from build123d import *

# Parameters (mm, degrees)
EXTRUSION1_DEPTH        = 21
ESQUISSE2_R             = 2.5
ENL_V_MAT_EXTRU_1_DEPTH = 22
ESQUISSE3_R             = 2.5
ENL_V_MAT_EXTRU_2_DEPTH = 40.5


with BuildPart() as part:
    # Esquisse1 → Extrusion1 (new body)
    with BuildSketch(Plane.XY):
        Polygon((0, -10.5), (0, 10.5), (9, 10.5), (9, 29), (34, 29), (34, 20), (14, 20), (14, -20), (34, -20), (34, -29), (9, -29), (9, -10.5), align=None)
    extrude(amount=EXTRUSION1_DEPTH)

    # Esquisse2 → Enlèv. mat.-Extru.1 (cut, through all)
    with BuildSketch(Plane.XY.offset(21)):
        with Locations((29, 24.5)):
            Circle(ESQUISSE2_R)
        with Locations((19, 24.5)):
            Circle(ESQUISSE2_R)
        with Locations((19, -24.5)):
            Circle(ESQUISSE2_R)
        with Locations((29, -24.5)):
            Circle(ESQUISSE2_R)
    extrude(amount=-ENL_V_MAT_EXTRU_1_DEPTH, mode=Mode.SUBTRACT)

    # Esquisse3 → Enlèv. mat.-Extru.2 (cut, through all)
    with BuildSketch(Plane(origin=(0, 10.5, 0), x_dir=(1, 0, 0), z_dir=(0, 1, 0))):
        with Locations((4.5, -5.5)):
            Circle(ESQUISSE3_R)
        with Locations((4.5, -15.5)):
            Circle(ESQUISSE3_R)
    extrude(amount=-ENL_V_MAT_EXTRU_2_DEPTH, mode=Mode.SUBTRACT)


solid = part.part
Could you check a few things on this model? Use its own coordinates, in mm. A direction names the side the tool comes from. Coordinates: 2 decimals unless noted, no trailing zeros. Loops run counter-clockwise (first coordinate to the right, second up) from the corner with the lowest first, then second, coordinate; pieces in that order, holes last. Notation, with made-up numbers: (-27, 9.5) -> (-8, 9.5) arc R19 ccw to (-8, 46.5) -> close; hole circle Ø6 at (49.5, -38). An arc over 180 degrees is marked (long way). Answer in a Markdown table with one row per item.
(1) For faces 5 (the face through (5, -10.5, 10)), 6 (the face through (4, 10.5, 10)), 7 (the face through (14, 0, 10)), which set-ups out of +Z, -Z, +X, -X, +Y, -Y let a thin tool reach every point of the face, with its end or its side?
Results found:
| item | result |
|---|---|
| face 5 | +Z, -Z, -X, -Y |
| face 6 | +Z, -Z, -X, +Y |
| face 7 | +Z, -Z, +X |
(2) Imagine slicing it at D-D (x = 23.5). List the corners of the cut face in (y, z) for me, plus the area to 3 significant figures.
Results found:
| item | result |
|---|---|
| outline | (-29, 0) -> (-20, 0) -> (-20, 21) -> (-29, 21) -> close; (20, 0) -> (29, 0) -> (29, 21) -> (20, 21) -> close |
| area | 378 mm^2 |
(3) Imagine slicing it at B-B (z = 15.5). List the corners of the cut face in (x, y) for me.
Results found:
| item | result |
|---|---|
| outline | (0, -10.5) -> (2, -10.5) -> (2, 10.5) -> (0, 10.5) -> close; (7, -10.5) -> (9, -10.5) -> (9, -29) -> (34, -29) -> (34, -20) -> (14, -20) -> (14, 20) -> (34, 20) -> (34, 29) -> (9, 29) -> (9, 10.5) -> (7, 10.5) -> close; hole circle Ø5 at (19, -24.5); hole circle Ø5 at (19, 24.5); hole circle Ø5 at (29, -24.5); hole circle Ø5 at (29, 24.5) |
(4) Imagine slicing it at C-C (x = 4.5). List the corners of the cut face in (y, z) for me.
Results found:
| item | result |
|---|---|
| outline | (-10.5, 0) -> (10.5, 0) -> (10.5, 3) -> (-10.5, 3) -> close; (-10.5, 8) -> (10.5, 8) -> (10.5, 13) -> (-10.5, 13) -> close; (-10.5, 18) -> (10.5, 18) -> (10.5, 21) -> (-10.5, 21) -> close |
(5) Thinking about a two-plate mould opening in Z: for faces 1 (the face through (6.81, 0.15, 16.46)), 2 (the face through (6.885, 0.147, 4.749)), 3 (the face through (24, -20, 10)), 4 (the face through (13, 2, 21)), which applies, released by +Z, released by -Z, zero draft, split by the parting line, or undercut?
Results found:
| item | result |
|---|---|
| face 1 | undercut |
| face 2 | undercut |
| face 3 | zero draft |
| face 4 | released by +Z |
(6) Will these pins go through, and if not, where does the flat tip stop? pin 1 Ø9 at (y, z) = (-23.5, 11.5) entering from -X; pin 2 Ø6 at (y, z) = (6, 2.5) entering from +X; pin 3 Ø4.5 at (x, z) = (5.5, 10) entering from +Y.
Results found:
| item | result |
|---|---|
| pin 1 | stops at x = 9 |
| pin 2 | stops at x = 14 |
| pin 3 | stops at y = 10.5 |
(7) If I drill on probe 1 along Y at (x, z) = (19, 7.25); probe 2 along X at (y, z) = (-24, 6.75); probe 3 along Y at (x, z) = (22, 17.25), over which ranges is the centre line in solid material (lowest first)?
Results found:
| item | result |
|---|---|
| probe 1 | y = -29 to -27, -22 to -20, 20 to 22, 27 to 29 |
| probe 2 | x = 9 to 16.55, 21.45 to 26.55, 31.45 to 34 |
| probe 3 | y = -29 to -20, 20 to 29 |
(8) Imagine slicing it at A-A (y = 24.5). List the corners of the cut face in (x, z) for me.
Results found:
| item | result |
|---|---|
| outline | (9, 0) -> (16.5, 0) -> (16.5, 21) -> (9, 21) -> close; (21.5, 0) -> (26.5, 0) -> (26.5, 21) -> (21.5, 21) -> close; (31.5, 0) -> (34, 0) -> (34, 21) -> (31.5, 21) -> close |
